CAD build for the part. Positions are in the model's coordinates, mm. Round coordinates to 2 decimals unless told otherwise and drop trailing zeros. Order: outer loops, then holes, each group sorted by start corner. A loop starts at its lowest first (then second) coordinate and runs counter-clockwise, first axis right, second up. Notation, with made-up numbers: (-2, 70) - (19, 70) arc R25 cw to (19, 105) - close; hole circle Ø5 at (-28.5, 2). An arc over 180 degrees is marked (long way). Write item = value, one per line.
from build123d import *

# Parameters (mm, degrees)
SKETCH1_W               = 115
SKETCH1_H               = 90
SKETCH1_R               = 1.65
BOSS_EXTRUDE2_DEPTH     = 7
CUT_EXTRUDE4_DEPTH      = 147.198495204
CUT_EXTRUDE4_DEPTH_BACK = 147.198495204
SKETCH5_R               = 1.65
FILLET1_R               = 5
SKETCH8_R               = 3.5
CUT_EXTRUDE6_DEPTH      = 4


with BuildPart() as part:
    # Sketch1 → Boss-Extrude2 (new body)
    with BuildSketch(Plane(origin=(0, 0, 0), x_dir=(1, 0, 0), z_dir=(0, 1, 0))):
        with Locations((57.5, 45)):
            Rectangle(SKETCH1_W, SKETCH1_H)
        with Locations(Location((10, 64.85, 0), (0, 0, 270))):
            Circle(SKETCH1_R, mode=Mode.SUBTRACT)
        with Locations(Location((31.4, 25.15, 0), (0, 0, 270))):
            Circle(SKETCH1_R, mode=Mode.SUBTRACT)
    extrude(amount=BOSS_EXTRUDE2_DEPTH)

    # Sketch5 → Cut-Extrude4 (cut, two sides: drawn at the far end of the back side and taken through both)
    with BuildSketch(Plane(origin=(0, 0, 0), x_dir=(-1, 0, 0), z_dir=(0, -1, 0)).offset(-CUT_EXTRUDE4_DEPTH_BACK)):
        with Locations(Location((-101, 17.4, 0), (0, 0, 90))):
            Circle(SKETCH5_R)
        with Locations(Location((-101, 72.6, 0), (0, 0, 90))):
            Circle(SKETCH5_R)
        with Locations(Location((-82, 17.4, 0), (0, 0, 90))):
            Circle(SKETCH5_R)
        with Locations(Location((-82, 72.6, 0), (0, 0, 90))):
            Circle(SKETCH5_R)
        with Locations(Location((-63, 17.4, 0), (0, 0, 90))):
            Circle(SKETCH5_R)
        with Locations(Location((-63, 72.6, 0), (0, 0, 90))):
            Circle(SKETCH5_R)
    extrude(amount=CUT_EXTRUDE4_DEPTH + CUT_EXTRUDE4_DEPTH_BACK, mode=Mode.SUBTRACT)

    # Fillet1
    fillet1_edges = [part.edges().sort_by_distance(p)[0] for p in [
        (0, 3.5, -90),
        (115, 3.5, -90),
        (115, 3.5, 0),
        (0, 3.5, 0),
    ]]
    fillet(fillet1_edges, radius=FILLET1_R)

    # Sketch8 → Cut-Extrude6 (cut)
    with BuildSketch(Plane.XZ):
        with Locations(Location((31.4, -25.15, 0), (0, 0, 270))):
            Circle(SKETCH8_R)
        with Locations(Location((10, -64.85, 0), (0, 0, 270))):
            Circle(SKETCH8_R)
        with Locations(Location((63, -72.6, 0), (0, 0, 270))):
            Circle(SKETCH8_R)
        with Locations(Location((82, -72.6, 0), (0, 0, 270))):
            Circle(SKETCH8_R)
        with Locations(Location((101, -72.6, 0), (0, 0, 270))):
            Circle(SKETCH8_R)
        with Locations(Location((63, -17.4, 0), (0, 0, 270))):
            Circle(SKETCH8_R)
        with Locations(Location((82, -17.4, 0), (0, 0, 270))):
            Circle(SKETCH8_R)
        with Locations(Location((101, -17.4, 0), (0, 0, 270))):
            Circle(SKETCH8_R)
    extrude(amount=-CUT_EXTRUDE6_DEPTH, mode=Mode.SUBTRACT)


solid = part.part
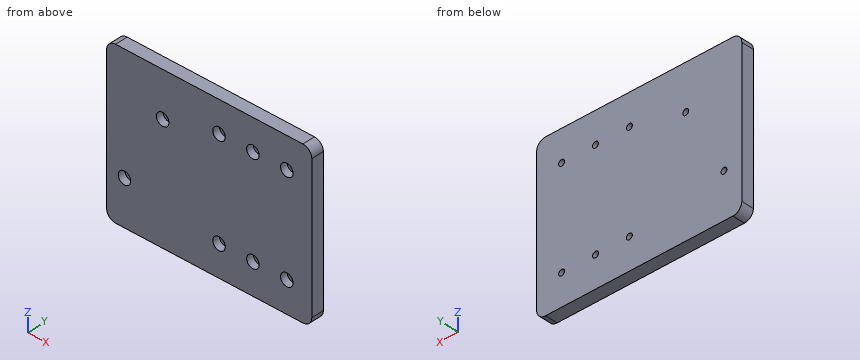
(1) Drop flat-ended pins along their axis: pin 1 (5.5 mm diameter, centred on x = 82, z = -72.6, fed in from -Y); pin 2 (11 mm diameter, centred on x = 63, z = -17.4, fed in from -Y). Give the stop position or say it passes through.
Solved:
pin_1 = 4
pin_2 = 0
(2) Probe line 1 along X through (y, z) = (1.9, -72.6); line 2 along X through (y, z) = (5.9, -72.6); line 3 along Z through (x, y) = (101, 5.8). List the from-to ranges inside material, lowest first.
Solved:
line_1 = 0 to 59.5, 66.5 to 78.5, 85.5 to 97.5, 104.5 to 115
line_2 = 0 to 61.35, 64.65 to 80.35, 83.65 to 99.35, 102.65 to 115
line_3 = -90 to -74.25, -70.95 to -19.05, -15.75 to 0
(3) Band-saw the part on A-A on x = 101. List the corners of the cut face in (y, z).
Solved:
outline = (0, -90) - (7, -90) - (7, -74.25) - (4, -74.25) - (4, -76.1) - (0, -76.1) - close; (0, -69.1) - (4, -69.1) - (4, -70.95) - (7, -70.95) - (7, -19.05) - (4, -19.05) - (4, -20.9) - (0, -20.9) - close; (0, -13.9) - (4, -13.9) - (4, -15.75) - (7, -15.75) - (7, 0) - (0, 0) - close
(4) Band-saw the part on C-C on y = 2.5. Count the separate pieces of the cut face and the enclosed holes in it, plus the area to 3 significant figures.
Solved:
separate_pieces = 1
enclosed_holes = 8
area = 10,000 mm²
(5) Band-saw the part on B-B on z = -64.85. List the corners of the cut face in (x, y).
Solved:
outline = (0, 0) - (6.5, 0) - (6.5, 4) - (8.35, 4) - (8.35, 7) - (0, 7) - close; (11.65, 4) - (13.5, 4) - (13.5, 0) - (115, 0) - (115, 7) - (11.65, 7) - close
(6) Band-saw the part on D-D on z = -17.4. List the corners of the cut face in (x, y), plus the area to 3 significant figures.
Solved:
outline = (0, 0) - (59.5, 0) - (59.5, 4) - (61.35, 4) - (61.35, 7) - (0, 7) - close; (64.65, 4) - (66.5, 4) - (66.5, 0) - (78.5, 0) - (78.5, 4) - (80.35, 4) - (80.35, 7) - (64.65, 7) - close; (83.65, 4) - (85.5, 4) - (85.5, 0) - (97.5, 0) - (97.5, 4) - (99.35, 4) - (99.35, 7) - (83.65, 7) - close; (102.65, 4) - (104.5, 4) - (104.5, 0) - (115, 0) - (115, 7) - (102.65, 7) - close
area = 691 mm²
